Could you check a few things on this model? Use its own coordinates, in mm. Face numbers are marked on the shaded views. Give positions to 0.01 mm unless a question says otherwise; leave off trailing zeros. Loops run counter-clockwise (first coordinate to the right, second up) from the corner with the lowest first, then second, coordinate; pieces in that order, holes last. Notation, with made-up numbers: M 24.5,-8.5 L 82.5,-8.5 A16 cw 82.5,20.5 Z; hole C 71,15 d1. An arc over 180 degrees is marked long. Return JSON: item names as keys, results as strings. Group by question number.
1. If we mould it in two halves opening along Z, with no side actions, what happens to the marked faces 1, 2, 3 and 4? For each: +Z half, -Z half, draft (parallel to the pull), parting line (faces both ways), or undercut.
2. Please list where these lines run through material, in increasing order: line 1 (Z direction, x = -1412.5, y = 680); line 2 (Y direction, x = -1417, z = -33.5); line 3 (X direction, y = 676, z = -28).
3. If we section it at C-C (z = 1): Write out the boundary of the cut face in (x, y), plus the area to 3 significant figures.
4. For pin 1 (5 mm diameter, centred on y = 700, z = 3.5, fed in from +X); pin 2 (4 mm diameter, centred on y = 686, z = -14.5, fed in from +X); pin 3 (0.5 mm diameter, centred on x = -1379.5, y = 655, fed in from -Z), each with a flat end and sliding along its axis, tell me the tip position at first contact or that it passes through.
5. If we section it at A-A (x = -1412): Write out the boundary of the cut face in (y, z).
6. If we section it at D-D (y = 681.5): Write out the boundary of the cut face in (x, z), plus the area to 3 significant figures.
7. If we section it at B-B (y = 672): Write out the boundary of the cut face in (x, z).
```python
from build123d import *

# Parameters (mm, degrees)
SKETCH1_R               = 6.00075
BOSS_EXTRUDE1_DEPTH     = 12.7
BOSS_EXTRUDE2_DEPTH     = 12.7
CUT_EXTRUDE1_DEPTH      = 26.4
CUT_EXTRUDE1_DEPTH_BACK = 26.4


with BuildPart() as part:
    # Sketch1 → Boss-Extrude1 (new body)
    with BuildSketch(Plane.XY):
        with BuildLine():
            Line((-1425.647832194, 709.279769852), (-1430.049287856, 669.182201206))
            ThreePointArc((-1430.049287856, 669.182201206), (-1425.788130872, 656.855717211), (-1413.552984482, 652.338986166))
            Line((-1413.552984482, 652.338986166), (-1371.063789142, 656.110020516))
            Line((-1371.063789142, 656.110020516), (-1425.647832194, 709.279769852))
        make_face()
        with Locations((-1414.900280944, 667.519315288)):
            Circle(SKETCH1_R, mode=Mode.SUBTRACT)
        with BuildLine():
            ThreePointArc((-1399.660280943, 667.519315289), (-1414.06759413, 682.736550014), (-1430.049287856, 669.182201206))
            ThreePointArc((-1430.049287856, 669.182201206), (-1429.244352574, 662.370994293), (-1425.534230405, 656.602506283))
            ThreePointArc((-1425.534230405, 656.602506283), (-1420.009574625, 653.161295993), (-1413.552984482, 652.338986166))
            ThreePointArc((-1413.552984482, 652.338986167), (-1403.657719001, 657.230369718), (-1399.660280943, 667.519315289))
        make_face()
        with Locations((-1414.900280944, 667.519315288)):
            Circle(SKETCH1_R, mode=Mode.SUBTRACT)
    boss_extrude1 = extrude(amount=BOSS_EXTRUDE1_DEPTH)

    # Sketch2 → Boss-Extrude2 (add, symmetric)
    with BuildSketch(Plane(origin=(0, 0, -12.7), x_dir=(-1, 0, 0), z_dir=(0, 0, -1))):
        Polygon((1422.066202071, 705.790941154), (1374.645419263, 659.598849213), (1379.65176797, 654.459333665), (1404.266329264, 678.436122134), (1427.072550778, 700.651425607), align=None)
    extrude(amount=BOSS_EXTRUDE2_DEPTH, both=True)

    # Mirror2: Boss-Extrude1 across plane
    add(boss_extrude1.mirror(Plane(origin=(0, 0, -12.7), x_dir=(1, 0, 0), z_dir=(0, 0, -1))))

    # Sketch4 → Cut-Extrude1 (cut, two sides)
    with BuildSketch(Plane(origin=(0, 0, -12.7), x_dir=(-1, 0, 0), z_dir=(0, 0, -1))) as cut_extrude1_sk:
        Polygon((1376.070137849, 650.970504969), (1371.063789142, 656.110020516), (1374.645419263, 659.598849213), (1379.65176797, 654.459333665), align=None)
        Polygon((1427.072550778, 700.651425607), (1430.654180901, 704.140254305), (1425.647832194, 709.279769852), (1422.066202071, 705.790941154), align=None)
    extrude(amount=CUT_EXTRUDE1_DEPTH, mode=Mode.SUBTRACT)
    extrude(cut_extrude1_sk.sketch, amount=-CUT_EXTRUDE1_DEPTH_BACK, mode=Mode.SUBTRACT)


solid = part.part
```
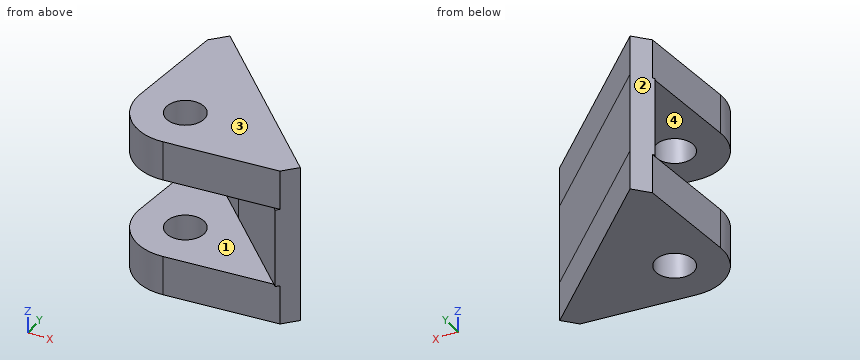
Answer:
{
 "1": {"face 1": "undercut", "face 2": "draft", "face 3": "+Z half", "face 4": "undercut"},
 "2": {"line 1": "z = -38.1 to -25.4, 0 to 12.7", "line 2": "y = 652.42 to 661.9, 673.14 to 700.86", "line 3": "x = -1429.3 to -1391.48"},
 "3": {"outline": "M -1430.05,669.18 A15.24 ccw -1413.55,652.34 L -1378.7,655.43 L -1374.65,659.6 L -1422.07,705.79 L -1426.53,701.2 Z; hole C -1414.9,667.52 d12", "area": "1,550 mm²"},
 "4": {"pin 1": "stops at x = -1413.55", "pin 2": "stops at x = -1399.7", "pin 3": "stops at z = -25.4"},
 "5": {"outline": "M 652.48,-38.1 L 662.27,-38.1 L 662.27,-25.4 L 652.48,-25.4 Z; M 652.48,0 L 662.27,0 L 662.27,12.7 L 652.48,12.7 Z; M 672.77,-38.1 L 695.99,-38.1 L 695.99,12.7 L 672.77,12.7 L 672.77,0 L 685.97,0 L 685.97,-25.4 L 672.77,-25.4 Z"},
 "6": {"outline": "M -1428.7,-38.1 L -1397.13,-38.1 L -1397.13,12.7 L -1428.7,12.7 L -1428.7,0 L -1407.41,0 L -1407.41,-25.4 L -1428.7,-25.4 Z", "area": "1,060 mm²"},
 "7": {"outline": "M -1429.74,-38.1 L -1418.89,-38.1 L -1418.89,-25.4 L -1429.74,-25.4 Z; M -1429.74,0 L -1418.89,0 L -1418.89,12.7 L -1429.74,12.7 Z; M -1410.91,-38.1 L -1387.38,-38.1 L -1387.38,12.7 L -1410.91,12.7 L -1410.91,0 L -1397.66,0 L -1397.66,-25.4 L -1410.91,-25.4 Z"}
}
